from build123d import *

# Parameters (mm, degrees)
EXTRUDE_1_DEPTH     = 5
SKETCH_8_OUTSIDE_W  = 22.464
SKETCH_8_OUTSIDE_H  = 20.522
SKETCH_8_OUTSIDE_R  = 6.278684177
CUT_EXTRUDE_1_DEPTH = 1
CUT_EXTRUDE_1_DRAFT = -45
SKETCH_9_R          = 3.825
BOLT_LENGTH_DEPTH   = 50
FILLET_1_R          = 1
CHAMFER_1_SIZE      = 1


with BuildPart() as part:
    # Эскиз6 → Бобышка-Вытянуть1 (new body)
    with BuildSketch(Plane(origin=(0, 0, 0), x_dir=(1, 0, 0), z_dir=(0, 1, 0))):
        Polygon((7.25, 0), (3.625, 6.278684177), (-3.625, 6.278684177), (-7.25, 0), (-3.625, -6.278684177), (3.625, -6.278684177), align=None)
    extrude(amount=EXTRUDE_1_DEPTH)


with BuildPart() as cut_extrude_1_tool:
    # Эскиз8 outside → Вырез-Вытянуть1 (with draft: the straight prism first)
    with BuildSketch(Plane(origin=(0, 5, 0), x_dir=(1, 0, 0), z_dir=(0, 1, 0))):
        Rectangle(SKETCH_8_OUTSIDE_W, SKETCH_8_OUTSIDE_H)
        Circle(SKETCH_8_OUTSIDE_R, mode=Mode.SUBTRACT)
    extrude(amount=-CUT_EXTRUDE_1_DEPTH)
    # Вырез-Вытянуть1: the draft: its side faces are tilted about the plane it starts from
    cut_extrude_1_sides = [cut_extrude_1_tool.faces().sort_by_distance(p)[0] for p in [
        (0, 4.5, 10.261),
        (11.232, 4.5, 0),
        (0, 4.5, -10.261),
        (-11.232, 4.5, 0),
        (-6.278684177, 4.5, 0),
    ]]
    draft(cut_extrude_1_sides, Plane(origin=(0, 5, 0), x_dir=(1, 0, 0), z_dir=(0, 1, 0)), CUT_EXTRUDE_1_DRAFT)


with BuildPart() as part_1:
    add(part.part)

    # Вырез-Вытянуть1: cut by cut_extrude_1_tool
    add(cut_extrude_1_tool.part, mode=Mode.SUBTRACT)

    # Эскиз9 → bolt length (add)
    with BuildSketch(Plane.XZ):
        with Locations(Location((0, 0, 0), (0, 0, 90))):  # turned: the seam where the file's is
            Circle(SKETCH_9_R)
    extrude(amount=BOLT_LENGTH_DEPTH)

    # Скругление1
    fillet_1_edges = [part_1.edges().sort_by_distance(p)[0] for p in [
        (0, 0, -3.825),
    ]]
    fillet(fillet_1_edges, radius=FILLET_1_R)

    # Фаска1
    chamfer_1_edges = [part_1.edges().sort_by_distance(p)[0] for p in [
        (0, -50, -3.825),
    ]]
    chamfer(chamfer_1_edges, length=CHAMFER_1_SIZE)


solid = part_1.part
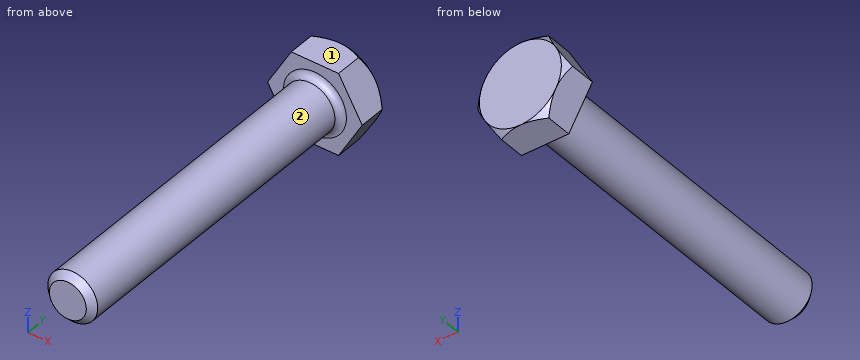
Model file for the job. Use its own axes, mm. Face numbers are marked on the shaded views. A direction names the side the tool comes from. Coordinates: 2 decimals unless noted, no trailing zeros. Write each loop counter-clockwise with the first axis right and the second up, starting at its lowest first coordinate (ties: lowest second). Pieces come first, ordered by that corner, then holes. Notation, with made-up numbers: (1.5, 33.25) - (12.5, 33.25) arc R25 ccw to (12.5, 47.25) - close; hole circle Ø5 at (41, 25.5). An arc over 180 degrees is marked (long way). Write each question's results on one line, items separated by ' | '. Start each with the question number.
1) Probe line 1 along Y through (x, z) = (-3.5, -4.25); line 2 along X through (y, z) = (-8, 3.5); line 3 along X through (y, z) = (-6.5, -1). List the from-to ranges inside material, lowest first. Write a range as from..to.
2) Cut at B-B (y = -20.5). Write the cut outline in (x, z) (3 decimals), then the cut area to 3 significant figures.
3) 3-axis set-ups, long thin cutter, end or side, ignore diameter. For the marked faces 1 and 2: which of +Z, -Z, +X, -X, +Y, -Y reach the whole face in a straight line?
4) Flat gauge pins, fed straight in: P1, Ø1, axis at x = -1, y = -37, coming from the +Z side; P2, Ø1, axis at y = -39.5, z = 3, coming from the +X side; P3, Ø4, axis at x = -3.5, y = -3.5, coming from the -Z side. Where does each tip first touch, or does it go through?
5) Cut at A-A (y = 0.5). Write the cut outline in (x, z) (3 decimals).
Returned:
1) line 1: 0..5 | line 2: -1.54..1.54 | line 3: -3.69..3.69
2) outline: circle Ø7.65 at (0, 0) | area: 46.0 mm^2
3) face 1: +Z, +X, -X, +Y, -Y | face 2: -Y
4) P1: z = 3.79 | P2: x = 2.89 | P3: z = -3.52
5) outline: (-7.25, 0) - (-3.625, -6.279) - (3.625, -6.279) - (7.25, 0) - (3.625, 6.279) - (-3.625, 6.279) - close
